The figure shows three views and two pictorial views of one solid part (mm, origin at its lowest corner). Answer the questions. A direction names the side the tool comes from. Round coordinates to 2 decimals unless told otherwise and drop trailing zeros. Order: outer loops, then holes, each group sorted by start corner. A loop starts at its lowest first (then second) coordinate and runs counter-clockwise, first axis right, second up. Notation, with made-up numbers: (46, 5.5) -> (97, 5.5) arc R27 ccw to (97, 28.5) -> close; hole circle Ø5 at (-35, -10). An arc over 180 degrees is marked (long way). One line per item, written item: value. Start each with the question number.
1. Section B-B (z = 4.25) is taken. Give the vertices of the cut face in (x, y).
2. For the marked faces 1, 2, 3, 4 and 5, determine the directions among +Z, -Z, +X, -X, +Y, -Y from which every point of the face is accessible in a straight line to the end or side of a thin tool.
3. Section A-A (x = 1.65) is taken. Give the vertices of the cut face in (y, z), then the cut area to 4 significant figures.
4. Section D-D (x = 46) is taken. Give the vertices of the cut face in (y, z).
5. Flat-ended cylindrical pins translate along their axes: pin 1 Ø6.5 at (x, z) = (51.5, 11.5) entering from +Y; pin 2 Ø5 at (y, z) = (17.5, 14.5) entering from -X; pin 3 Ø3 at (x, z) = (3.5, 5.5) entering from -Y. Find the tip coordinate at first contact, or state that the pin passes through.
6. Consider line 1 (Z direction, x = 51, y = 29); line 2 (Y direction, x = 24, z = 11); line 3 (X direction, y = 21, z = 10.5). Determine where each line is inside the solid, lowest interval first.
7. Section C-C (y = 6) is taken. Give the vertices of the cut face in (x, z), then the cut area to 3 significant figures.
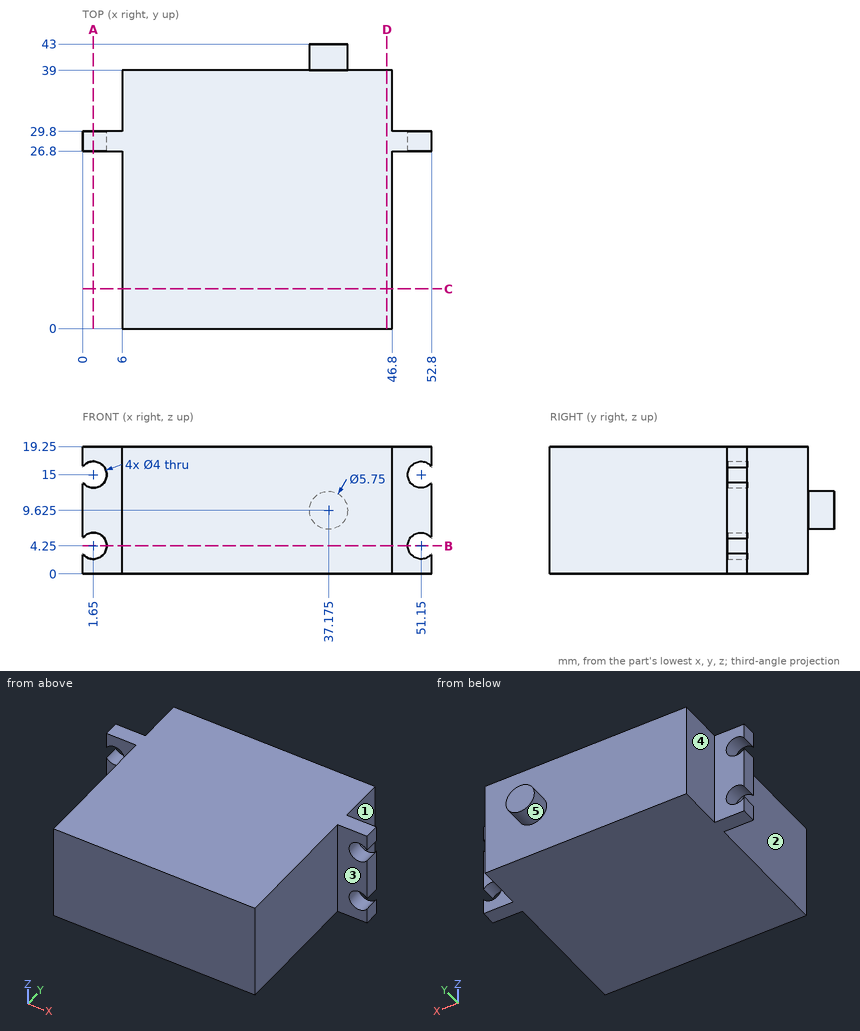
Answer:
1. outline: (3.65, 26.8) -> (6, 26.8) -> (6, 0) -> (46.8, 0) -> (46.8, 26.8) -> (49.15, 26.8) -> (49.15, 29.8) -> (46.8, 29.8) -> (46.8, 39) -> (6, 39) -> (6, 29.8) -> (3.65, 29.8) -> close
2. face 1: +Z, -Z, +X, +Y
2. face 2: +Z, -Z, -X, -Y
2. face 3: +Z, -Z, +X, -Y
2. face 4: +Z, -Z, -X, +Y
2. face 5: +Y
3. outline: (26.8, 0) -> (29.8, 0) -> (29.8, 2.25) -> (26.8, 2.25) -> close; (26.8, 6.25) -> (29.8, 6.25) -> (29.8, 13) -> (26.8, 13) -> close; (26.8, 17) -> (29.8, 17) -> (29.8, 19.25) -> (26.8, 19.25) -> close
3. area: 33.75 mm^2
4. outline: (0, 0) -> (39, 0) -> (39, 19.25) -> (0, 19.25) -> close
5. pin 1: y = 29.8
5. pin 2: x = 6
5. pin 3: y = 26.8
6. line 1: 0 to 2.26, 6.24 to 13.01, 16.99 to 19.25
6. line 2: 0 to 39
6. line 3: 6 to 46.8
7. outline: (6, 0) -> (46.8, 0) -> (46.8, 19.25) -> (6, 19.25) -> close
7. area: 785 mm^2
